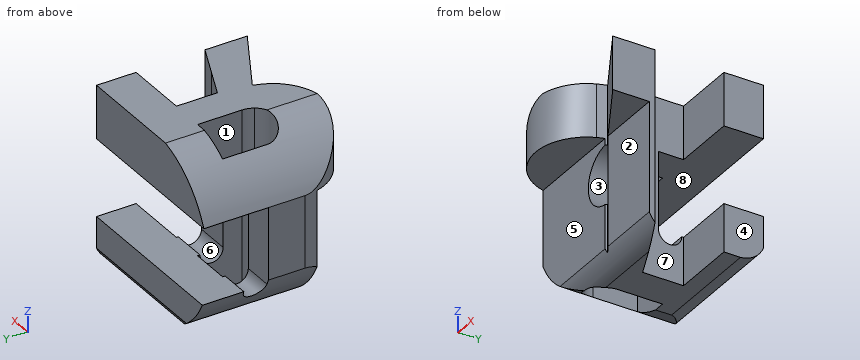
from build123d import *

# Parameters (mm, degrees)
F0_W     = 50
F0_H     = 50
F1_DEPTH = 50
F3_DEPTH = 50.001
F5_DEPTH = 50.001
F7_DEPTH = 50.001


# Not quite as in the source:
# - a feature names something its author has since deleted; it is built from what else it names


with BuildPart() as f1:
    # F0 (on Top) → F1 (new body)
    with BuildSketch(Plane.XY):
        Rectangle(F0_W, F0_H)
    extrude(amount=F1_DEPTH)

    # F2 (on face) → F3 (cut, through all)
    with BuildSketch(Plane(origin=(0, 25, 0), x_dir=(-1, 0, 0), z_dir=(0, 1, 0))):
        with BuildLine():
            ThreePointArc((-6.6122752614, 16.6977748275), (2.2958755953, 25), (-6.6122752614, 33.3022251725))
            Line((-6.6122752614, 33.3022251725), (-6.6122752614, 16.6977748275))
        make_face()
        with BuildLine():
            ThreePointArc((5.8814799413, 50), (19.5641723767, 41.0564068722), (25, 25.640320846))
            Line((25, 25.640320846), (25, 50))
            Line((25, 50), (5.8814799413, 50))
        make_face()
        with BuildLine():
            Line((25, 0), (25, 24.359679154))
            ThreePointArc((25, 24.359679154), (19.5641723767, 8.9435931278), (5.8814799413, 0))
            Line((5.8814799413, 0), (25, 0))
        make_face()
    extrude(amount=-F3_DEPTH, mode=Mode.SUBTRACT)

    # F4 (on face) → F5 (cut, through all)
    with BuildSketch(Plane.YZ.offset(25)):
        Polygon((-6.9390782155, 35.097297281), (-25, 35.097297281), (-25, 0), (-6.9390782155, 0), (-6.9390782155, 4.401256796), (-6.9390782155, 13.4532200173), align=None)
        with BuildLine():
            Line((25, 13.4532200173), (25, 35.097297281))
            Line((25, 35.097297281), (6.9390782155, 35.097297281))
            Line((6.9390782155, 35.097297281), (6.9390782155, 13.4532200173))
            ThreePointArc((6.9390782155, 13.4532200173), (10.1754756179, 10.2168226149), (13.4118730202, 13.4532200173))
            Line((13.4118730202, 13.4532200173), (25, 13.4532200173))
        make_face()
        with BuildLine():
            Line((25, 0), (25, 4.6294564381))
            ThreePointArc((25, 4.6294564381), (22.4439231862, 1.4056456338), (18.5773167759, 0))
            Line((18.5773167759, 0), (25, 0))
        make_face()
        with BuildLine():
            Line((-6.9390782155, 4.401256796), (-6.9390782155, 0))
            Line((-6.9390782155, 0), (-1.2912911565, 0))
            ThreePointArc((-1.2912911565, 0), (-4.7087911569, 1.438899851), (-6.9390782155, 4.401256796))
        make_face()
    extrude(amount=-F5_DEPTH, mode=Mode.SUBTRACT)

    # F6 (on face) → F7 (cut, through all)
    with BuildSketch(Plane(origin=(0, 0, 0), x_dir=(1, 0, 0), z_dir=(0, 0, -1))):
        Polygon((-27.4569652975, -12.0541369542), (-23.0521892468, -12.0541369542), (-23.0521892468, 3.30411084), (-23.0521892468, 9.0968515724), (-27.4569652975, 9.0968515724), align=None)
        Polygon((6.9360537454, -13.9329824597), (25, -13.9329824597), (25, 1.2912911565), (15.6700833973, 1.2912911565), (6.9360537454, -2.4867046159), align=None)
        with BuildLine():
            Line((-23.0521892468, 9.0968515724), (-23.0521892468, 3.30411084))
            ThreePointArc((-23.0521892468, 3.30411084), (-11.5730780457, 17.3836701729), (4.5299022458, 8.9754592627))
            Line((4.5299022458, 8.9754592627), (5.442249123, 6.361215841))
            Line((5.442249123, 6.361215841), (25, 17.1625725925))
            Line((25, 17.1625725925), (25, 25))
            Line((25, 25), (-23.0521892468, 25))
            Line((-23.0521892468, 25), (-23.0521892468, 9.0968515724))
        make_face()
        Polygon((15.6700833973, 1.2912911565), (25, 1.2912911565), (25, 5.3270440549), align=None)
        with BuildLine():
            Line((-5.8814799413, 1.2912911565), (-5.8814799413, -14.1096981242))
            Line((-5.8814799413, -14.1096981242), (-2.7823168784, -14.1096981242))
            Line((-2.7823168784, -14.1096981242), (-2.7823168784, -1.6426106449))
            ThreePointArc((-2.7823168784, -1.6426106449), (-2.9925352611, -0.1187433848), (-3.6074871188, 1.2912911565))
            Line((-3.6074871188, 1.2912911565), (-5.8814799413, 1.2912911565))
        make_face()
        with BuildLine():
            Line((-14.0390070155, -14.1096981242), (-5.8814799413, -14.1096981242))
            Line((-5.8814799413, -14.1096981242), (-5.8814799413, 1.2912911565))
            Line((-5.8814799413, 1.2912911565), (-3.6074871188, 1.2912911565))
            ThreePointArc((-3.6074871188, 1.2912911565), (-9.9345292071, 3.7755160409), (-14.0390070155, -1.6426106449))
            Line((-14.0390070155, -1.6426106449), (-14.0390070155, -14.1096981242))
        make_face()
    extrude(amount=-F7_DEPTH, mode=Mode.SUBTRACT)


solid = f1.part
Could you check a few things on this model? Use its own coordinates, in mm. Face numbers are marked on the shaded views. A direction names the side the tool comes from. Round coordinates to 2 decimals unless told otherwise and drop trailing zeros. Write each loop counter-clockwise with the first axis right and the second up, starting at its lowest first coordinate (ties: lowest second). Pieces come first, ordered by that corner, then holes. Notation, with made-up numbers: (30, 61) -> (36, 61) arc R21 cw to (36, 81) -> close; hole circle Ø3 at (19.5, 49.25). An arc over 180 degrees is marked (long way). Use a Markdown table: item, result.
1. If we section it at A-A (z = 25): List the corners of the cut face in (x, y) for me, then the cut area to 3 significant figures.
Answer key:
| item | result |
|---|---|
| outline | (-23.05, -3.3) arc R14.37 ccw to (-22.58, -6.94) -> (-2.3, -6.94) -> (-2.3, 6.94) -> (-2.78, 6.94) -> (-2.78, 1.64) arc R5.63 cw to (-14.04, 1.64) -> (-14.04, 6.94) -> (-23.05, 6.94) -> close; (6.61, -6.94) -> (25, -6.94) -> (25, -5.33) -> (6.94, 2.49) -> (6.94, 6.94) -> (6.61, 6.94) -> close |
| area | 282 mm^2 |
2. If we section it at B-B (y = -2): List the corners of the cut face in (x, z) for me.
Answer key:
| item | result |
|---|---|
| outline | (-23.05, 14.9) arc R25.49 ccw to (-12.7, 2.87) -> (-12.7, 47.13) arc R25.49 ccw to (-23.05, 35.1) -> close; (-4.12, 0.13) -> (17.31, 0.13) -> (17.31, 50) -> (-4.12, 50) -> close; hole (6.61, 16.7) -> (6.61, 33.3) arc R8.32 ccw (long way) to start |
3. For pin 1 Ø5.5 at (y, z) = (5.5, 15.5) entering from +X; pin 2 Ø14 at (x, z) = (-3.5, 20) entering from -Y; pin 3 Ø8 at (x, z) = (4.5, 19.5) entering from +Y, each with a flat end and sliding along its axis, tell me the tip position at first contact or that it passes through.
Answer key:
| item | result |
|---|---|
| pin 1 | stops at x = 6.94 |
| pin 2 | stops at y = -6.94 |
| pin 3 | stops at y = 6.94 |
4. We'd pull the mould along X, two halves only. Please class the marked faces 1, 2, 3 and 4: +X half, -X half, draft (parallel to the pull), parting line (faces both ways), or undercut.
Answer key:
| item | result |
|---|---|
| face 1 | undercut |
| face 2 | draft |
| face 3 | undercut |
| face 4 | +X half |
5. Please list where these lines run through material, in increasing order: probe 1 along Y at (x, z) = (23, 45); probe 2 along Z at (x, y) = (-15.5, 10.5); probe 3 along Y at (x, z) = (-12.5, 42).
Answer key:
| item | result |
|---|---|
| probe 1 | y = -16.06 to -4.46, 13.93 to 25 |
| probe 2 | z = 4.83 to 10.23, 35.1 to 45.17 |
| probe 3 | y = -17.16 to -2.22, 14.11 to 25 |
6. Which directions (+Z, -Z, +X, -X, +Y, -Y) give clear straight access to the entire face, cutting with the end or side of a thin tool? Please do the marked faces 5, 6, 7 and 8.
Answer key:
| item | result |
|---|---|
| face 5 | -Z, +X, -X, -Y |
| face 6 | +X, -X |
| face 7 | +Z, -Z, +X |
| face 8 | +X, -X, +Y |
7. If we section it at C-C (x = 14): List the corners of the cut face in (y, z) for me.
Answer key:
| item | result |
|---|---|
| outline | (-11.09, 35.1) -> (-6.94, 35.1) -> (-6.94, 4.4) arc R7.12 ccw to (-1.29, 0) -> (-0.57, 0) -> (-0.57, 50) -> (-11.09, 50) -> close; (13.93, 0) -> (18.58, 0) arc R7.55 ccw to (25, 4.63) -> (25, 13.45) -> (13.93, 13.45) -> close; (13.93, 35.1) -> (25, 35.1) -> (25, 50) -> (13.93, 50) -> close |
8. If we section it at D-D (y = -8): List the corners of the cut face in (x, z) for me, then the cut area to 3 significant figures.
Answer key:
| item | result |
|---|---|
| outline | (-22.26, 35.1) -> (4.87, 35.1) -> (4.87, 50) -> (-5.88, 50) arc R25.49 ccw to (-22.26, 36.81) -> close; (8.41, 35.1) -> (25, 35.1) -> (25, 50) -> (8.41, 50) -> close |
| area | 576 mm^2 |
